from build123d import *

# Parameters (mm, degrees)
SKETCH1_W       = 23.2
SKETCH1_H       = 31.2
BEZEL_DEPTH     = 2.5
SKETCH2_W       = 14
SKETCH2_H       = 22
ROCKER_DEPTH    = 5.5
SKETCH3_W       = 21.6
SKETCH3_H       = 29.6
BODY_DEPTH      = 24
SKETCH4_W       = 12
SKETCH4_H       = 20
TERMINALS_DEPTH = 8


with BuildPart() as part:
    # Sketch1 → Bezel (new body)
    with BuildSketch(Plane.XY):
        Rectangle(SKETCH1_W, SKETCH1_H)
    extrude(amount=BEZEL_DEPTH)

    # Sketch2 → Rocker (add)
    with BuildSketch(Plane.XY.offset(2.5)):
        Rectangle(SKETCH2_W, SKETCH2_H)
    extrude(amount=ROCKER_DEPTH)

    # Sketch3 → Body (add)
    with BuildSketch(Plane.XY.offset(-24)):
        Rectangle(SKETCH3_W, SKETCH3_H)
    extrude(amount=BODY_DEPTH)

    # Sketch4 → Terminals (add)
    with BuildSketch(Plane.XY.offset(-32)):
        Rectangle(SKETCH4_W, SKETCH4_H)
    extrude(amount=TERMINALS_DEPTH)


solid = part.part
Design review of the part built by this model. Coordinates are the model's own, in mm. A direction names the side the tool comes from. Round coordinates to 2 decimals unless told otherwise and drop trailing zeros. Loops run counter-clockwise (first coordinate to the right, second up) from the corner with the lowest first, then second, coordinate; pieces in that order, holes last. Notation, with made-up numbers: M -31,72 L -17,72 A22 cw -17,97 Z; hole C 10.5,-7.5 d1. An arc over 180 degrees is marked long. Answer as a JSON object with one key per item and string values.
Item 1: We need section D-D on x = -9.75. Give the boundary of the cut face in (y, z), and give its area (3 significant figures).
Answer sheet:
{"outline": "M -15.6,0 L -14.8,0 L -14.8,-24 L 14.8,-24 L 14.8,0 L 15.6,0 L 15.6,2.5 L -15.6,2.5 Z", "area": "788 mm^2"}
Item 2: We need section A-A on x = -1. Give the boundary of the cut face in (y, z).
Answer sheet:
{"outline": "M -15.6,0 L -14.8,0 L -14.8,-24 L -10,-24 L -10,-32 L 10,-32 L 10,-24 L 14.8,-24 L 14.8,0 L 15.6,0 L 15.6,2.5 L 11,2.5 L 11,8 L -11,8 L -11,2.5 L -15.6,2.5 Z"}
Item 3: We need section B-B on y = -13. Give the boundary of the cut face in (x, z), and give its area (3 significant figures).
Answer sheet:
{"outline": "M -11.6,0 L -10.8,0 L -10.8,-24 L 10.8,-24 L 10.8,0 L 11.6,0 L 11.6,2.5 L -11.6,2.5 Z", "area": "576 mm^2"}
Item 4: We need section C-C on z = -3.5. Give the boundary of the cut face in (x, y), and give its area (3 significant figures).
Answer sheet:
{"outline": "M -10.8,-14.8 L 10.8,-14.8 L 10.8,14.8 L -10.8,14.8 Z", "area": "639 mm^2"}
Item 5: Wall thickness on L1, parallel to Y at x = -6, z = -19; L2, parallel to Y at x = 2.5, z = 6; L3, parallel to X at y = 10.5, z = -12.5: over which ranges is each line inside the solid? List them lowest first. Write a range as from..to.
Answer sheet:
{"L1": "y = -14.8..14.8", "L2": "y = -11..11", "L3": "x = -10.8..10.8"}
Item 6: Clearance check with flat-ended pins moving along their axes: P1, Ø7, axis at y = -1.5, z = -16, coming from the +X side; P2, Ø1, axis at x = -7, y = 9.5, coming from the -Z side; P3, Ø6, axis at x = 0, z = 4.5, coming from the -Y side; P4, Ø9, axis at y = 2.5, z = -29, coming from the -X side. State where each tip first meets the part, or that it passes through.
Answer sheet:
{"P1": "stops at x = 10.8", "P2": "stops at z = -24", "P3": "stops at y = -15.6", "P4": "stops at x = -6"}
Item 7: Machinability: for faces 1 (the flat face through (0, -10, -28)), 2 (the flat face through (6, 0, -28)), 3 (the flat face through (-6, 0, -28)), 4 (the flat face through (0, -11, 5)), which of the approach directions +Z, -Z, +X, -X, +Y, -Y give a long, thin tool a straight path to every point of the face, cutting with its end or side? Answer none if there is none.
Answer sheet:
{"face 1": "-Z, +X, -X, -Y", "face 2": "-Z, +X, +Y, -Y", "face 3": "-Z, -X, +Y, -Y", "face 4": "+Z, +X, -X, -Y"}
